from build123d import *

# Parameters (mm, degrees)
F0_W     = 40
F0_H     = 22
F1_DEPTH = 3
F2_R     = 3
F3_DEPTH = 0.5
F4_R     = 2.4
F5_DEPTH = 3.5
F6_R     = 3.75
F7_DEPTH = 25


with BuildPart() as f1:
    # F0 (on Front) → F1 (new body)
    with BuildSketch(Plane.XZ):
        with Locations((20, 11)):
            Rectangle(F0_W, F0_H)
    extrude(amount=F1_DEPTH)

    # F2 (on face) → F3 (join)
    with BuildSketch(Plane.XZ.offset(3)):
        with Locations((20, 11)):
            Circle(F2_R)
    extrude(amount=F3_DEPTH)

    # F4 (on face) → F5 (join)
    with BuildSketch(Plane.XZ.offset(3.5)):
        with Locations((20, 11)):
            Circle(F4_R)
    extrude(amount=F5_DEPTH)

    # F6 (on face) → F7 (cut)
    with BuildSketch(Plane.XZ.offset(3)):
        with Locations((5, 11)):
            Circle(F6_R)
        with Locations((35, 11)):
            Circle(F6_R)
    extrude(amount=-F7_DEPTH, mode=Mode.SUBTRACT)


solid = f1.part
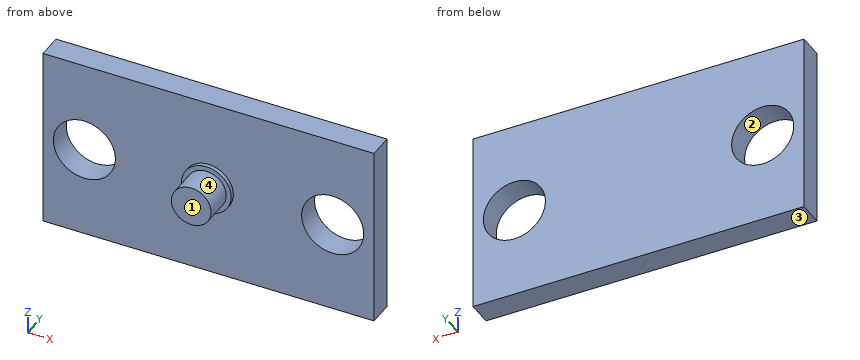
Check sheet for the modelled part. Datum: model origin and axes. Units: mm. Face numbers are marked on the shaded views. Round coordinates to 2 decimals unless told otherwise and drop trailing zeros. Write each loop counter-clockwise with the first axis right and the second up, starting at its lowest first coordinate (ties: lowest second). Pieces come first, ordered by that corner, then holes. Notation, with made-up numbers: (54.5, 19) -> (75.5, 19) arc R19 ccw to (75.5, 49) -> close; hole circle Ø5 at (10.25, 31.5). An arc over 180 degrees is marked (long way). Answer as CSV lines item,"result". Start each with the question number.
1) Material ranges on line 1 (Z direction, x = 5, y = -1.65); line 2 (Y direction, x = 11.5, z = 8.25); line 3 (Z direction, x = 33.5, y = -0.75), recorded low to high. Write a range as from..to.
2) Release check for a two-part mould opening along Z. For the marked faces 1, 2, 3 and 4 record: pulls with the +Z half, pulls with the -Z half, needs draft (parallel to the pull), parting line crosses it, or undercut.
3) Section check C-C on y = -1.25. Enter the section's corners in (x, z).
4) Go/stop test with flat-tipped pins: P1, Ø4, axis at x = 24.5, z = 19.5, coming from the -Y side; P2, Ø2, axis at x = 6, z = 10.5, coming from the -Y side; P3, Ø1.5, axis at y = -6, z = 9.5, coming from the +X side. Record where each tip stops, or that it passes through.
5) Section check A-A on x = 35. Enter the section's corners in (y, z).
6) Section check D-D on x = 20. Enter the section's corners in (y, z).
7) Section check B-B on z = 10. Enter the section's corners in (x, y).
Found:
1,line 1,"z = 0..7.25, 14.75..22"
1,line 2,"y = -3..0"
1,line 3,"z = 0..7.56, 14.44..22"
2,face 1,"needs draft"
2,face 2,"undercut"
2,face 3,"pulls with the -Z half"
2,face 4,"parting line crosses it"
3,outline,"(0, 0) -> (40, 0) -> (40, 22) -> (0, 22) -> close; hole circle Ø7.5 at (5, 11); hole circle Ø7.5 at (35, 11)"
4,P1,"stops at y = -3"
4,P2,"passes through"
4,P3,"stops at x = 22.28"
5,outline,"(-3, 0) -> (0, 0) -> (0, 7.25) -> (-3, 7.25) -> close; (-3, 14.75) -> (0, 14.75) -> (0, 22) -> (-3, 22) -> close"
6,outline,"(-7, 8.6) -> (-3.5, 8.6) -> (-3.5, 8) -> (-3, 8) -> (-3, 0) -> (0, 0) -> (0, 22) -> (-3, 22) -> (-3, 14) -> (-3.5, 14) -> (-3.5, 13.4) -> (-7, 13.4) -> close"
7,outline,"(0, -3) -> (1.39, -3) -> (1.39, 0) -> (0, 0) -> close; (8.61, -3) -> (17.17, -3) -> (17.17, -3.5) -> (17.82, -3.5) -> (17.82, -7) -> (22.18, -7) -> (22.18, -3.5) -> (22.83, -3.5) -> (22.83, -3) -> (31.39, -3) -> (31.39, 0) -> (8.61, 0) -> close; (38.61, -3) -> (40, -3) -> (40, 0) -> (38.61, 0) -> close"
